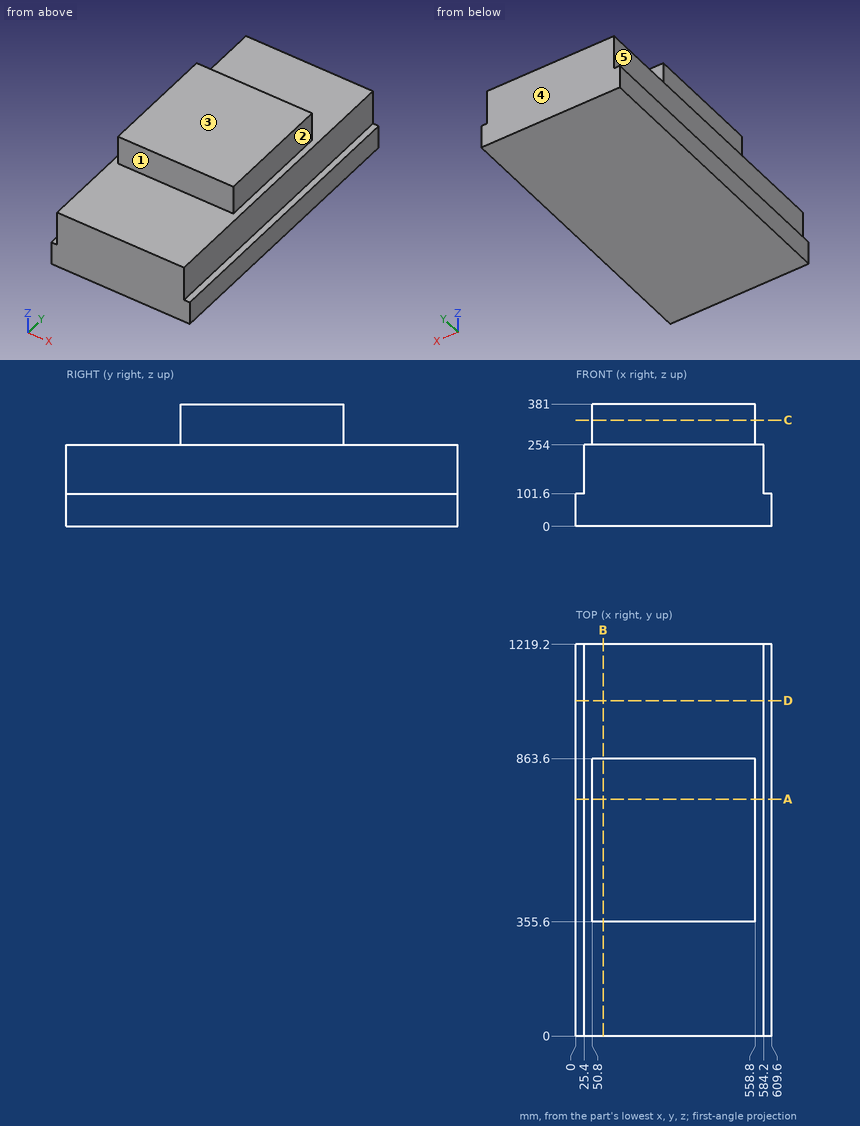
Input: dimensioned drawing with shaded views. Units: mm. Origin: part minimum x, y, z. A direction names the side the tool comes from. Round coordinates to 2 decimals unless told otherwise and drop trailing zeros. Write each loop counter-clockwise with the first axis right and the second up, starting at its lowest first coordinate (ties: lowest second). Pieces come first, ordered by that corner, then holes. Notation, with made-up numbers: (3, -27.5) -> (16, -27.5) arc R4 cw to (16, -21.5) -> close; hole circle Ø6 at (32.25, 5.5). An arc over 180 degrees is marked (long way). Use CSV: the item, a comma, the result in double quotes. Start each with the question number.
Q1. Section B-B (x = 85). Return loops of the section in (y, z).
Q2. Section C-C (z = 330.5). Return loops of the section in (x, y), plus the area to 3 significant figures.
Q3. Section A-A (y = 737.5). Return loops of the section in (x, z), plus the area to 3 significant figures.
Q4. Section D-D (y = 1044). Return loops of the section in (x, z).
Q5. First-contact query: pin 1 Ø8 at (y, z) = (1073.5, 174.5) entering from -X; pin 2 Ø3 at (y, z) = (719, 238) entering from +X; pin 3 Ø2 at (x, z) = (316, 275) entering from +Y. Flat tips, straight axial feed; report the tip coordinate or a pass-through.
Q6. Reachability of the marked faces 1, 2, 3, 4 and 5 from +Z, -Z, +X, -X, +Y, -Y: full face, straight path, thin tool, end or side. Return the list, or none.
Q7. Line query: L1, parallel to Y at x = 522, z = 275.5; L2, parallel to Z at x = 50.5, y = 443.5; L3, parallel to X at y = 493, z = 259. Output: solid intervals per line, ascending.
Result sheet:
1,outline,"(0, 0) -> (1219.2, 0) -> (1219.2, 254) -> (863.6, 254) -> (863.6, 381) -> (355.6, 381) -> (355.6, 254) -> (0, 254) -> close"
2,outline,"(50.8, 355.6) -> (558.8, 355.6) -> (558.8, 863.6) -> (50.8, 863.6) -> close"
2,area,"258,000 mm²"
3,outline,"(0, 0) -> (609.6, 0) -> (609.6, 101.6) -> (584.2, 101.6) -> (584.2, 254) -> (558.8, 254) -> (558.8, 381) -> (50.8, 381) -> (50.8, 254) -> (25.4, 254) -> (25.4, 101.6) -> (0, 101.6) -> close"
3,area,"212,000 mm²"
4,outline,"(0, 0) -> (609.6, 0) -> (609.6, 101.6) -> (584.2, 101.6) -> (584.2, 254) -> (25.4, 254) -> (25.4, 101.6) -> (0, 101.6) -> close"
5,pin 1,"x = 25.4"
5,pin 2,"x = 584.2"
5,pin 3,"y = 863.6"
6,face 1,"+Z, +X, -X, -Y"
6,face 2,"+Z, +X, +Y, -Y"
6,face 3,"+Z, +X, -X, +Y, -Y"
6,face 4,"+Z, -Z, +X, -X, +Y"
6,face 5,"+Z, -X, +Y, -Y"
7,L1,"355.6 to 863.6"
7,L2,"0 to 254"
7,L3,"50.8 to 558.8"
